Check sheet for the modelled part. Datum: model origin and axes. Units: mm. Face numbers are marked on the shaded views. A direction names the side the tool comes from. Give positions to 0.01 mm unless a question says otherwise; leave off trailing zeros. Order: outer loops, then holes, each group sorted by start corner. A loop starts at its lowest first (then second) coordinate and runs counter-clockwise, first axis right, second up.
Item 1: Sectioned sample at D-D on z = 1.5. Record the boundary of the cut face in (x, y), and give its area (3 significant figures).
Item 2: Material ranges on line 1 along Y through (x, z) = (0.1, 8.2); line 2 along X through (y, z) = (-12.25, 0.5), recorded low to high.
Item 3: Sectioned sample at A-A on z = 5.75. Record the boundary of the cut face in (x, y).
Item 4: Gauge pin test, flat ends, axial feed: P1, Ø0.8, axis at x = -4.5, z = 9, coming from the -Y side; P2, Ø2, axis at x = 9, y = 1.5, coming from the -Z side; P3, Ø0.8, axis at y = 10, z = 8.5, coming from the +X side. Record the tip position at first contact, or that the pin passes through.
Item 5: Sectioned sample at B-B on x = 0.1. Record the boundary of the cut face in (y, z), and give its area (3 significant figures).
Item 6: Access from +Z, -Z, +X, -X, +Y, -Y to the whole of each face (thin tool, end or side, straight path). Record for the marked faces 1 and 2.
Item 7: Release check for a two-part mould opening along X. For the marked faces 3, 4 and 5 record: released by +X, released by -X, zero draft, split by the parting line, or undercut.
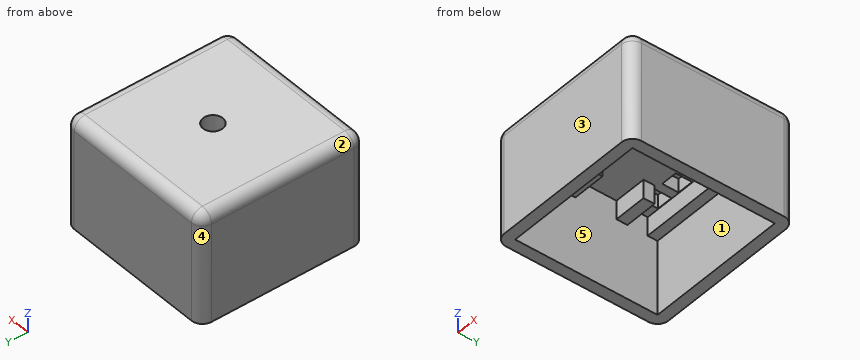
from build123d import *

# Parameters (mm, degrees)
CYLINDER001_R     = 1.8
CYLINDER001_DEPTH = 3
BOX006_W          = 3
BOX006_H          = 3
BOX006_DEPTH      = 3
BOX005_W          = 3
BOX005_H          = 3
BOX005_DEPTH      = 3
BOX003_W          = 3
BOX003_H          = 3
BOX003_DEPTH      = 3
BOX004_W          = 3
BOX004_H          = 3
BOX004_DEPTH      = 3
BOX002_W          = 3
BOX002_H          = 3
BOX002_DEPTH      = 3
BOX_W             = 26
BOX_H             = 26
BOX_DEPTH         = 17
BOX001_W          = 30
BOX001_H          = 30
BOX001_DEPTH      = 20
BOX010_W          = 6
BOX010_H          = 2
BOX010_DEPTH      = 3.4
BOX008_W          = 4
BOX008_H          = 4
BOX008_DEPTH      = 3.4
BOX007_W          = 26
BOX007_H          = 1.8
BOX007_DEPTH      = 3.4
BOX009_W          = 6
BOX009_H          = 2
BOX009_DEPTH      = 3.4
BOX011_W          = 6
BOX011_H          = 2
BOX011_DEPTH      = 3.4
FILLET_R          = 2


with BuildPart() as obj1:
    # Cylinder001 → Cylinder001 (new body)
    with BuildSketch(Plane(origin=(0.1, 0.3, 7), x_dir=(1, 0, 0), z_dir=(0, 0, 1))):
        Circle(CYLINDER001_R)
    extrude(amount=CYLINDER001_DEPTH)


with BuildPart() as l5:
    # Box006 → Box006 (new body)
    with BuildSketch(Plane(origin=(7.67, 8.11, 6.5), x_dir=(1, 0, 0), z_dir=(0, 0, 1))):
        with Locations((1.5, 1.5)):
            Rectangle(BOX006_W, BOX006_H)
    extrude(amount=BOX006_DEPTH)


with BuildPart() as l4:
    # Box005 → Box005 (new body)
    with BuildSketch(Plane(origin=(3.1, 8.11, 6.5), x_dir=(1, 0, 0), z_dir=(0, 0, 1))):
        with Locations((1.5, 1.5)):
            Rectangle(BOX005_W, BOX005_H)
    extrude(amount=BOX005_DEPTH)


with BuildPart() as l2:
    # Box003 → Box003 (new body)
    with BuildSketch(Plane(origin=(-6.04, 8.11, 6.5), x_dir=(1, 0, 0), z_dir=(0, 0, 1))):
        with Locations((1.5, 1.5)):
            Rectangle(BOX003_W, BOX003_H)
    extrude(amount=BOX003_DEPTH)


with BuildPart() as l3:
    # Box004 → Box004 (new body)
    with BuildSketch(Plane(origin=(-1.47, 8.11, 6.5), x_dir=(1, 0, 0), z_dir=(0, 0, 1))):
        with Locations((1.5, 1.5)):
            Rectangle(BOX004_W, BOX004_H)
    extrude(amount=BOX004_DEPTH)


with BuildPart() as fusion:
    # Box002 → Box002 (new body)
    with BuildSketch(Plane(origin=(-10.61, 8.11, 6.5), x_dir=(1, 0, 0), z_dir=(0, 0, 1))):
        with Locations((1.5, 1.5)):
            Rectangle(BOX002_W, BOX002_H)
    extrude(amount=BOX002_DEPTH)

    # Fusion: union L5, L4, L2, L3
    add(l5.part)
    add(l4.part)
    add(l2.part)
    add(l3.part)


with BuildPart() as maininside:
    # Box → Box (new body)
    with BuildSketch(Plane(origin=(-13, -13, -10), x_dir=(1, 0, 0), z_dir=(0, 0, 1))):
        with Locations((13, 13)):
            Rectangle(BOX_W, BOX_H)
    extrude(amount=BOX_DEPTH)


with BuildPart() as cut002:
    # Box001 → Box001 (new body)
    with BuildSketch(Plane(origin=(-15, -15, -10), x_dir=(1, 0, 0), z_dir=(0, 0, 1))):
        with Locations((15, 15)):
            Rectangle(BOX001_W, BOX001_H)
    extrude(amount=BOX001_DEPTH)

    # Cut: cut MainInside
    add(maininside.part, mode=Mode.SUBTRACT)

    # Cut001: cut Fusion
    add(fusion.part, mode=Mode.SUBTRACT)

    # Cut002: cut obj1
    add(obj1.part, mode=Mode.SUBTRACT)


with BuildPart() as obj2:
    # Box010 → Box010 (new body)
    with BuildSketch(Plane(origin=(-13, 5.5, 3.6), x_dir=(1, 0, 0), z_dir=(0, 0, 1))):
        with Locations((3, 1)):
            Rectangle(BOX010_W, BOX010_H)
    extrude(amount=BOX010_DEPTH)


with BuildPart() as obj3:
    # Box008 → Box008 (new body)
    with BuildSketch(Plane(origin=(8, 0, 3.6), x_dir=(1, 0, 0), z_dir=(0, 0, 1))):
        with Locations((2, 2)):
            Rectangle(BOX008_W, BOX008_H)
    extrude(amount=BOX008_DEPTH)


with BuildPart() as obj4:
    # Box007 → Box007 (new body)
    with BuildSketch(Plane(origin=(-13, 11.2, 3.6), x_dir=(1, 0, 0), z_dir=(0, 0, 1))):
        with Locations((13, 0.9)):
            Rectangle(BOX007_W, BOX007_H)
    extrude(amount=BOX007_DEPTH)


with BuildPart() as obj5:
    # Box009 → Box009 (new body)
    with BuildSketch(Plane(origin=(-13, -4, 3.6), x_dir=(1, 0, 0), z_dir=(0, 0, 1))):
        with Locations((3, 1)):
            Rectangle(BOX009_W, BOX009_H)
    extrude(amount=BOX009_DEPTH)


with BuildPart() as fillet_body:
    # Box011 → Box011 (new body)
    with BuildSketch(Plane(origin=(7, -13, 3.6), x_dir=(1, 0, 0), z_dir=(0, 0, 1))):
        with Locations((3, 1)):
            Rectangle(BOX011_W, BOX011_H)
    extrude(amount=BOX011_DEPTH)

    # Fusion002: union obj2, obj3, obj4, obj5
    add(obj2.part)
    add(obj3.part)
    add(obj4.part)
    add(obj5.part)

    # Fusion005: union Cut002
    add(cut002.part)

    # Fillet
    fillet_edges = [fillet_body.edges().sort_by_distance(p)[0] for p in [
        (-15, 0, 10),
        (0, 15, 10),
        (0, -15, 10),
        (15, 0, 10),
        (-15, -15, 0),
        (-15, 15, 0),
        (15, 15, 0),
        (15, -15, 0),
    ]]
    fillet(fillet_edges, radius=FILLET_R)


solid = fillet_body.part
Report:
1. outline: (-15, -13) arc R2 ccw to (-13, -15) - (13, -15) arc R2 ccw to (15, -13) - (15, 13) arc R2 ccw to (13, 15) - (-13, 15) arc R2 ccw to (-15, 13) - close; hole (-13, -13) - (13, -13) - (13, 13) - (-13, 13) - close
1. area: 221 mm2
2. line 1: y = -14.99 to -1.5, 2.1 to 8.11, 11.11 to 14.99
2. line 2: x = -15 to -13, 13 to 15
3. outline: (-15, -13) arc R2 ccw to (-13, -15) - (13, -15) arc R2 ccw to (15, -13) - (15, 13) arc R2 ccw to (13, 15) - (-13, 15) arc R2 ccw to (-15, 13) - close; (8, 0) - (12, 0) - (12, 4) - (8, 4) - close; hole (-13, -13) - (7, -13) - (7, -11) - (13, -11) - (13, 11.2) - (-13, 11.2) - (-13, 7.5) - (-7, 7.5) - (-7, 5.5) - (-13, 5.5) - (-13, -2) - (-7, -2) - (-7, -4) - (-13, -4) - close
4. P1: stops at y = -14.91
4. P2: stops at z = 3.6
4. P3: stops at x = 15
5. outline: (-15, -10) - (-13, -10) - (-13, 7) - (-1.5, 7) - (-1.5, 10) - (-13, 10) arc R2 ccw to (-15, 8) - close; (2.1, 7) - (8.11, 7) - (8.11, 9.5) - (11.11, 9.5) - (11.11, 7) - (11.2, 7) - (11.2, 3.6) - (13, 3.6) - (13, -10) - (15, -10) - (15, 8) arc R2 ccw to (13, 10) - (2.1, 10) - close
5. area: 144 mm2
6. face 1: -Z
6. face 2: +Z, -X, +Y, -Y
7. face 3: zero draft
7. face 4: released by -X
7. face 5: undercut
